```python
from build123d import *

# Parameters (mm, degrees)
BOSS_EXTRUDE1_DEPTH      = 190.5
BOSS_EXTRUDE1_DEPTH_BACK = 190.5
SKETCH2_W                = 381
SKETCH2_H                = 6.35
BOSS_EXTRUDE2_DEPTH      = 25.4
SKETCH3_R                = 3.96875
CUT_EXTRUDE1_DEPTH       = 25.4
SKETCH4_R                = 3.937
CUT_EXTRUDE2_DEPTH       = 302.34078715


with BuildPart() as part:
    # Sketch1 → Boss-Extrude1 (new, two sides: drawn at the far end of the back side and taken through both)
    with BuildSketch(Plane(origin=(0, 0, 0), x_dir=(0, 0, -1), z_dir=(1, 0, 0)).offset(-BOSS_EXTRUDE1_DEPTH_BACK)):
        with BuildLine():
            Line((-139.7, 0), (139.7, 0))
            ThreePointArc((139.7, 0), (193.581536726, 22.318463274), (215.9, 76.2))
            Line((215.9, 76.2), (203.2, 76.2))
            ThreePointArc((203.2, 76.2), (184.601280605, 31.298719395), (139.7, 12.7))
            Line((139.7, 12.7), (-139.7, 12.7))
            Line((-139.7, 12.7), (-139.7, 0))
        make_face()
    extrude(amount=BOSS_EXTRUDE1_DEPTH + BOSS_EXTRUDE1_DEPTH_BACK)

    # Sketch2 → Boss-Extrude2 (add)
    with BuildSketch(Plane(origin=(0, 76.2, 0), x_dir=(1, 0, 0), z_dir=(0, 1, 0))):
        with Locations((0, 206.375)):
            Rectangle(SKETCH2_W, SKETCH2_H)
    extrude(amount=BOSS_EXTRUDE2_DEPTH)

    # Sketch3 → Cut-Extrude1 (cut)
    with BuildSketch(Plane(origin=(0, 0, -209.55), x_dir=(-1, 0, 0), z_dir=(0, 0, -1))):
        with Locations((-139.7, 88.9)):
            Circle(SKETCH3_R)
        with Locations((139.7, 88.9)):
            Circle(SKETCH3_R)
        with Locations((0, 88.9)):
            Circle(SKETCH3_R)
    extrude(amount=-CUT_EXTRUDE1_DEPTH, mode=Mode.SUBTRACT)

    # Sketch4 → Cut-Extrude2 (cut, through all)
    with BuildSketch(Plane(origin=(0, 12.7, 0), x_dir=(1, 0, 0), z_dir=(0, 1, 0))):
        with Locations(Location((176.784, -101.6, 0), (0, 0, 270))):
            Circle(SKETCH4_R)
        with Locations(Location((176.784, 101.6, 0), (0, 0, 270))):
            Circle(SKETCH4_R)
        with Locations(Location((-176.784, -101.6, 0), (0, 0, 90))):
            Circle(SKETCH4_R)
        with Locations(Location((-176.784, 101.6, 0), (0, 0, 90))):
            Circle(SKETCH4_R)
    extrude(amount=-CUT_EXTRUDE2_DEPTH, mode=Mode.SUBTRACT)


solid = part.part
```
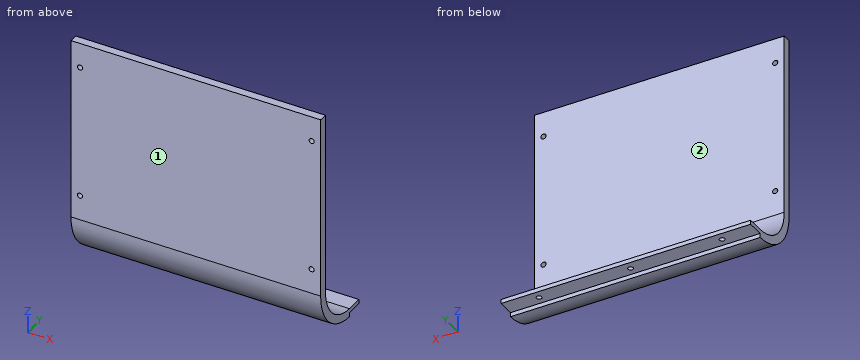
Source: CAD feature listing. Evaluate the final solid. Frame: model axes, mm. Face numbers are marked on the shaded views. A direction names the side the tool comes from. Give positions to 0.01 mm unless a question says otherwise; leave off trailing zeros. Order: outer loops, then holes, each group sorted by start corner. A loop starts at its lowest first (then second) coordinate and runs counter-clockwise, first axis right, second up.
(1) Access query for the marked faces 1 and 2. Directions: +Z, -Z, +X, -X, +Y, -Y. A direction counts if a zero-diameter tool reaches every point of the face in a straight line with its end or side. Return the directions, or none.
(2) Material intervals for line 1 along X through (y, z) = (8, -101.6); line 2 along X through (y, z) = (4, -101); line 3 along Y through (x, z) = (166, -92), sorted ascending.
(3) Section query C-C (y = 69.5). Return the cut outline in (x, z).
(4) Section query A-A (x = 152). Return the cut outline in (y, z), plus the area to 3 significant figures.
(5) Contact query for flat-ended pins moving along their axis: P1, Ø10, axis at x = -3.5, y = 12.5, coming from the -Z side; P2, Ø12, axis at x = 77, y = 36, coming from the -Z side; P3, Ø12.5, axis at x = 176.784, z = 101.6, coming from the +Y side. Output: stop coordinate, or through.
(6) Section query B-B (z = -57.5). Return the cut outline in (x, y).
Outcome:
1. face 1: +Z, -Z, +X, -X, -Y
1. face 2: +Z, +X, -X, +Y
2. line 1: x = -190.5 to -180.72, -172.85 to 172.85, 180.72 to 190.5
2. line 2: x = -190.5 to -180.68, -172.89 to 172.89, 180.68 to 190.5
2. line 3: y = 0 to 12.7
3. outline: (-190.5, -215.6) - (190.5, -215.6) - (190.5, -202.85) - (-190.5, -202.85) - close
4. outline: (0, -139.7) arc R76.2 ccw to (76.2, -215.9) - (76.2, -209.55) - (101.6, -209.55) - (101.6, -203.2) - (76.2, -203.2) arc R63.5 cw to (12.7, -139.7) - (12.7, 139.7) - (0, 139.7) - close
4. area: 5,100 mm2
5. P1: stops at z = -188.29
5. P2: stops at z = -207.79
5. P3: stops at y = 12.7
6. outline: (-190.5, 0) - (190.5, 0) - (190.5, 12.7) - (-190.5, 12.7) - close
